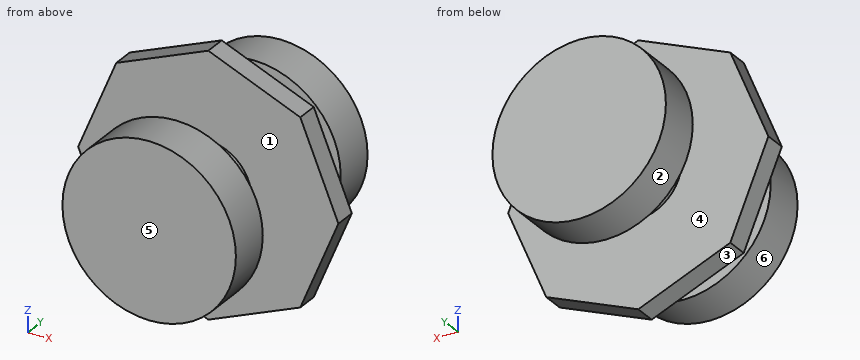
```python
from build123d import *

# Parameters (mm, degrees)
SKETCH2_R           = 20
BOSS_EXTRUDE1_DEPTH = 10
SKETCH3_R           = 10
BOSS_EXTRUDE2_DEPTH = 12
BOSS_EXTRUDE3_DEPTH = 5
SKETCH5_R           = 10
BOSS_EXTRUDE4_DEPTH = 12
SKETCH6_R           = 20
BOSS_EXTRUDE5_DEPTH = 10


with BuildPart() as part:
    # Sketch2 → Boss-Extrude1 (new body)
    with BuildSketch(Plane(origin=(0, 0, 0), x_dir=(1, 0, 0), z_dir=(0, 1, 0))):
        with Locations(Location((0, 0, 0), (0, 0, 270))):
            Circle(SKETCH2_R)
    extrude(amount=BOSS_EXTRUDE1_DEPTH)

    # Sketch3 → Boss-Extrude2 (add)
    with BuildSketch(Plane(origin=(0, 10, 0), x_dir=(1, 0, 0), z_dir=(0, 1, 0))):
        with Locations(Location((0, 0, 0), (0, 0, 270))):
            Circle(SKETCH3_R)
    extrude(amount=BOSS_EXTRUDE2_DEPTH)

    # Sketch4 → Boss-Extrude3 (add)
    with BuildSketch(Plane(origin=(0, 22, 0), x_dir=(1, 0, 0), z_dir=(0, 1, 0))):
        Polygon((30, 0), (21.213203436, 21.213203436), (0, 30), (-21.213203436, 21.213203436), (-30, 0), (-21.213203436, -21.213203436), (0, -30), (21.213203436, -21.213203436), align=None)
    extrude(amount=BOSS_EXTRUDE3_DEPTH)

    # Sketch5 → Boss-Extrude4 (add)
    with BuildSketch(Plane(origin=(0, 27, 0), x_dir=(1, 0, 0), z_dir=(0, 1, 0))):
        with Locations(Location((0, 0, 0), (0, 0, 270))):
            Circle(SKETCH5_R)
    extrude(amount=BOSS_EXTRUDE4_DEPTH)

    # Sketch6 → Boss-Extrude5 (add)
    with BuildSketch(Plane(origin=(0, 39, 0), x_dir=(1, 0, 0), z_dir=(0, 1, 0))):
        with Locations(Location((0, 0, 0), (0, 0, 270))):
            Circle(SKETCH6_R)
    extrude(amount=BOSS_EXTRUDE5_DEPTH)


solid = part.part
```
Model file for the job. Use its own axes, mm. Face numbers are marked on the shaded views. A direction names the side the tool comes from. Round coordinates to 2 decimals unless told otherwise and drop trailing zeros. Write each loop counter-clockwise with the first axis right and the second up, starting at its lowest first coordinate (ties: lowest second). Pieces come first, ordered by that corner, then holes. Notation, with made-up numbers: (52, 21) - (101, 21) arc R23 cw to (101, 35) - close; hole circle Ø5 at (16, 12). An arc over 180 degrees is marked (long way). One line per item, written item: value.
(1) Cut at A-A, the plane y = 24.5. Give the cut face in (x, z).
Values follow:
outline: (-30, 0) - (-21.21, -21.21) - (0, -30) - (21.21, -21.21) - (30, 0) - (21.21, 21.21) - (0, 30) - (-21.21, 21.21) - close
(2) Cut at B-B, the plane x = 12.5. Give the cut face in (y, z), plus the area to 3 significant figures.
Values follow:
outline: (0, -15.61) - (10, -15.61) - (10, 15.61) - (0, 15.61) - close; (22, -24.82) - (27, -24.82) - (27, 24.82) - (22, 24.82) - close; (39, -15.61) - (49, -15.61) - (49, 15.61) - (39, 15.61) - close
area: 873 mm²
(3) Two-plate mould, pull along Y, no slides. Class the marked faces 4, 5 and 6: pulls with the +Y half, pulls with the -Y half, needs draft (parallel to the pull), parting line crosses it, or undercut.
Values follow:
face 4: undercut
face 5: pulls with the -Y half
face 6: needs draft
(4) Drop flat-ended pins along their axis: P1, Ø3, axis at x = 22, z = -21, coming from the -Y side; P2, Ø4, axis at y = 37, z = -23, coming from the -X side; P3, Ø8, axis at x = -22, z = 23, coming from the +Y side; P4, Ø2, axis at x = 14.5, y = 23.5, coming from the -Z side. Give the stop position or say it passes through.
Values follow:
P1: stops at y = 22
P2: passes through
P3: stops at y = 27
P4: stops at z = -24.41
(5) Wall check: probe 1 along Y at (x, z) = (17, -7); probe 2 along Y at (x, z) = (-14, 17); probe 3 along Z at (x, y) = (-11, 47). Give the ranges that are in metal, low to high.
Values follow:
probe 1: y = 0 to 10, 22 to 27, 39 to 49
probe 2: y = 22 to 27
probe 3: z = -16.7 to 16.7
(6) Cut at C-C, the plane z = -11.5. Give the cut face in (x, y), plus the area to 3 significant figures.
Values follow:
outline: (-25.24, 22) - (25.24, 22) - (25.24, 27) - (-25.24, 27) - close; (-16.36, 0) - (16.36, 0) - (16.36, 10) - (-16.36, 10) - close; (-16.36, 39) - (16.36, 39) - (16.36, 49) - (-16.36, 49) - close
area: 907 mm²
(7) Cut at D-D, the plane x = 2. Give the cut face in (y, z).
Values follow:
outline: (0, -19.9) - (10, -19.9) - (10, -9.8) - (22, -9.8) - (22, -29.17) - (27, -29.17) - (27, -9.8) - (39, -9.8) - (39, -19.9) - (49, -19.9) - (49, 19.9) - (39, 19.9) - (39, 9.8) - (27, 9.8) - (27, 29.17) - (22, 29.17) - (22, 9.8) - (10, 9.8) - (10, 19.9) - (0, 19.9) - close
(8) 3-axis set-ups, long thin cutter, end or side, ignore diameter. For the marked faces 1, 2 and 3: which of +Z, -Z, +X, -X, +Y, -Y reach the whole face in a straight line?
Values follow:
face 1: none
face 2: +Y
face 3: -Z, -X, +Y, -Y
